The listing builds one solid part. Answer for the finished solid, in the listing's coordinates (mm). A direction names the side the tool comes from. Give positions to 0.01 mm unless a question says otherwise; leave off trailing zeros. Write each loop counter-clockwise with the first axis right and the second up, starting at its lowest first coordinate (ties: lowest second). Pieces come first, ordered by that corner, then holes. Notation, with made-up numbers: (-10, 44) -> (33, 44) arc R29 cw to (33, 82) -> close; hole circle Ø1 at (-24.5, -29). An arc over 180 degrees is marked (long way). Put each result on its own line as item: value. Start each with the question number.
1) For faces 1 (the flat face through (-25, -31, 1)), 2 (the flat face through (-21, -37, 1)), determine the directions among +Z, -Z, +X, -X, +Y, -Y from which every point of the face is accessible in a straight line to the end or side of a thin tool.
2) A cutting plane is placed at D-D (y = 17.5). Write down the section's boundary in (x, z), then the cut area to 3 significant figures.
3) Find the intervals of material crossed by line 1 along Y through (x, z) = (-26, 0.5); line 2 along X through (y, z) = (-16, 1.4); line 3 along X through (y, z) = (-1.5, 1.35), in increasing order. Write a range as from..to.
4) A cutting plane is placed at A-A (x = -24). Write down the section's boundary in (y, z), then the cut area to 3 significant figures.
5) A cutting plane is placed at C-C (x = -5). Write down the section's boundary in (y, z).
6) For a pull along Y with two mould halves and no side action, classify faces 3 (the flat face through (-25, -22.75, 1)), 4 (the cylindrical face through (-1.141, 35.797, 1.014)), 5 (the flat face through (-23, -18.25, 1)), 6 (the flat face through (0, 0, 1)) as released by +Y, released by -Y, zero draft, split by the parting line, or undercut.
from build123d import *

# Parameters (mm, degrees)
SKETCH_1_R      = 2
EXTRUDE_1_DEPTH = 2
FILLET_1_R      = 4


with BuildPart() as part:
    # ｽｹｯﾁ1 → ﾎﾞｽ - 押し出し1 (new body)
    with BuildSketch(Plane.XY):
        Polygon((-38, -31), (-38, -37), (0, -37), (0, 37), (-38, 37), (-38, 31), (-8, 31), (-8, 22.75), (-38, 22.75), (-38, 18.25), (-8, 18.25), (-8, 10.3), (-38, 10.3), (-38, 4.3), (-8, 4.3), (-8, -4.3), (-38, -4.3), (-38, -10.3), (-8, -10.3), (-8, -18.25), (-38, -18.25), (-38, -22.75), (-8, -22.75), (-8, -31), align=None)
        with Locations((-4, 0)):
            Circle(SKETCH_1_R, mode=Mode.SUBTRACT)
    extrude(amount=EXTRUDE_1_DEPTH)

    # ﾌｨﾚｯﾄ1
    fillet_1_edges = [part.edges().sort_by_distance(p)[0] for p in [
        (-8, -31, 1),
        (-8, -22.75, 1),
        (-8, -4.3, 1),
        (-8, 4.3, 1),
        (-8, 22.75, 1),
        (-8, 31, 1),
        (0, 37, 1),
        (0, -37, 1),
    ]]
    fillet(fillet_1_edges, radius=FILLET_1_R)


solid = part.part
Reply:
1. face 1: +Z, -Z, -X
1. face 2: +Z, -Z, +X, -X, -Y
2. outline: (-8, 0) -> (0, 0) -> (0, 2) -> (-8, 2) -> close
2. area: 16.0 mm2
3. line 1: y = -37..-31, -22.75..-18.25, -10.3..-4.3, 4.3..10.3, 18.25..22.75, 31..37
3. line 2: x = -8..0
3. line 3: x = -8.18..-5.32, -2.68..0
4. outline: (-37, 0) -> (-31, 0) -> (-31, 2) -> (-37, 2) -> close; (-22.75, 0) -> (-18.25, 0) -> (-18.25, 2) -> (-22.75, 2) -> close; (-10.3, 0) -> (-4.3, 0) -> (-4.3, 2) -> (-10.3, 2) -> close; (4.3, 0) -> (10.3, 0) -> (10.3, 2) -> (4.3, 2) -> close; (18.25, 0) -> (22.75, 0) -> (22.75, 2) -> (18.25, 2) -> close; (31, 0) -> (37, 0) -> (37, 2) -> (31, 2) -> close
4. area: 66.0 mm2
5. outline: (-37, 0) -> (-1.73, 0) -> (-1.73, 2) -> (-37, 2) -> close; (1.73, 0) -> (37, 0) -> (37, 2) -> (1.73, 2) -> close
6. face 3: undercut
6. face 4: released by +Y
6. face 5: undercut
6. face 6: zero draft
